```python
from build123d import *

# Parameters (mm, degrees)
BOSS_EXTRUDE1_DEPTH  = 10
M3_CLEARANCE_HOLE1_D = 3.4


with BuildPart() as part:
    # Sketch2 → Boss-Extrude1 (new body)
    with BuildSketch(Plane.XY):
        with BuildLine():
            Line((12.5, 0), (17.5, 0))
            Line((17.5, 0), (17.5, 17.5))
            Line((17.5, 17.5), (-17.5, 17.5))
            Line((-17.5, 17.5), (-17.5, 0))
            Line((-17.5, 0), (-12.5, 0))
            ThreePointArc((-12.5, 0), (0, 12.5), (12.5, 0))
        make_face()
    extrude(amount=BOSS_EXTRUDE1_DEPTH)

    # M3 Clearance Hole1 (through all)
    with Locations(Plane(origin=(0, 17.5, 0), x_dir=(1, 0, 0), z_dir=(0, 1, 0))):
        with Locations((-15, -5), (15, -5)):
            Hole(M3_CLEARANCE_HOLE1_D / 2)


solid = part.part
```
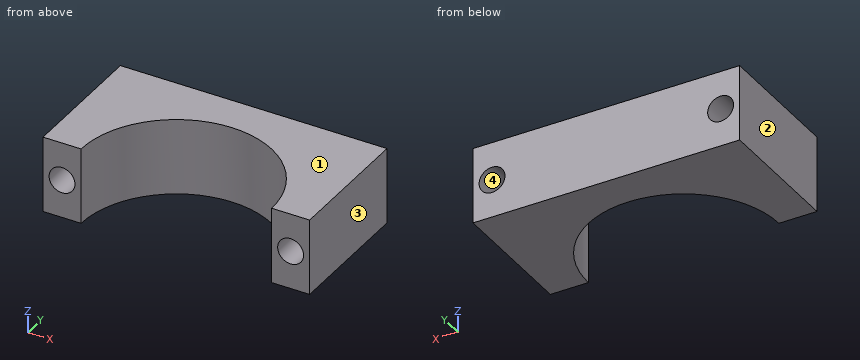
Geometry check sheet. Reference: the model listing, model coordinates, mm. Face numbers are marked on the shaded views. Give positions to 0.01 mm unless a question says otherwise; leave off trailing zeros. Write each loop counter-clockwise with the first axis right and the second up, starting at its lowest first coordinate (ties: lowest second). Pieces come first, ordered by that corner, then holes. Notation, with made-up numbers: (2, 3) - (33, 3) arc R22 cw to (33, 25) - close; hole circle Ø11 at (-12.5, -14). An arc over 180 degrees is marked (long way). Use a Markdown table: item, result.
Q1. Draft check along X on the marked faces 1, 2, 3 and 4. Enter one of: pulls with the +X half, pulls with the -X half, needs draft (parallel to the pull), parting line crosses it, or undercut.
Computed:
| item | result |
|---|---|
| face 1 | needs draft |
| face 2 | pulls with the -X half |
| face 3 | pulls with the +X half |
| face 4 | undercut |
Q2. Section check A-A, the plane x = -15. Enter the section's corners in (y, z), then the cut area to 4 significant figures.
Computed:
| item | result |
|---|---|
| outline | (0, 0) - (17.5, 0) - (17.5, 3.3) - (0, 3.3) - close; (0, 6.7) - (17.5, 6.7) - (17.5, 10) - (0, 10) - close |
| area | 115.5 mm² |
Q3. Section check D-D, the plane y = 16. Enter the section's corners in (x, z).
Computed:
| item | result |
|---|---|
| outline | (-17.5, 0) - (17.5, 0) - (17.5, 10) - (-17.5, 10) - close; hole circle Ø3.4 at (-15, 5); hole circle Ø3.4 at (15, 5) |
Q4. Go/stop test with a flat-tipped pin: P1, Ø4, axis at x = 9, z = 5, coming from the -Y side. Record where the tip stops, or that it passes through.
Computed:
| item | result |
|---|---|
| P1 | stops at y = 5.94 |
Q5. Section check B-B, the plane y = 5. Enter the section's corners in (x, z), then the cut area to 3 significant figures.
Computed:
| item | result |
|---|---|
| outline | (-17.5, 0) - (-11.46, 0) - (-11.46, 10) - (-17.5, 10) - close; (11.46, 0) - (17.5, 0) - (17.5, 10) - (11.46, 10) - close; hole circle Ø3.4 at (-15, 5); hole circle Ø3.4 at (15, 5) |
| area | 103 mm² |
Q6. Thickness scan on L1, parallel to X at y = 12.75, z = 5; L2, parallel to X at y = 4, z = 5; L3, parallel to X at y = 7.5, z = 5. Record the ranges inside material, lowest first. Write a range as [from, to].
Computed:
| item | result |
|---|---|
| L1 | x = [-17.5, -16.7], [-13.3, 13.3], [16.7, 17.5] |
| L2 | x = [-17.5, -16.7], [-13.3, -11.84], [11.84, 13.3], [16.7, 17.5] |
| L3 | x = [-17.5, -16.7], [-13.3, -10], [10, 13.3], [16.7, 17.5] |
Q7. Section check C-C, the plane z = 5. Enter the section's corners in (x, y).
Computed:
| item | result |
|---|---|
| outline | (-17.5, 0) - (-16.7, 0) - (-16.7, 17.5) - (-17.5, 17.5) - close; (-13.3, 0) - (-12.5, 0) arc R12.5 cw to (12.5, 0) - (13.3, 0) - (13.3, 17.5) - (-13.3, 17.5) - close; (16.7, 0) - (17.5, 0) - (17.5, 17.5) - (16.7, 17.5) - close |
